from build123d import *

# Parameters (mm, degrees)
ESQUISSE1_W             = 30
ESQUISSE1_H             = 290
BOSS_EXTRU_1_DEPTH      = 5
ESQUISSE1_6_W           = 5
ESQUISSE1_6_H           = 8
ENL_V_MAT_EXTRU_1_DEPTH = 5
ESQUISSE1_7_W           = 5
ESQUISSE1_7_H           = 15
ESQUISSE1_7_H_2         = 8
ENL_V_MAT_EXTRU_2_DEPTH = 5


with BuildPart() as part:
    # Esquisse1 → Boss.-Extru.1 (new body)
    with BuildSketch(Plane.XY):
        with Locations((-15, 145)):
            Rectangle(ESQUISSE1_W, ESQUISSE1_H)
    extrude(amount=BOSS_EXTRU_1_DEPTH)

    # Esquisse1<6> → Enlèv. mat.-Extru.1 (cut)
    with BuildSketch(Plane.XY):
        with Locations((-2.5, 286)):
            Rectangle(ESQUISSE1_6_W, ESQUISSE1_6_H)
    extrude(amount=ENL_V_MAT_EXTRU_1_DEPTH, mode=Mode.SUBTRACT)

    # Esquisse1<7> → Enlèv. mat.-Extru.2 (cut)
    with BuildSketch(Plane.XY):
        with Locations((-21.11, 25)):
            Rectangle(ESQUISSE1_7_W, ESQUISSE1_7_H)
        with Locations((-21.11, 83)):
            Rectangle(ESQUISSE1_7_W, ESQUISSE1_7_H)
        with Locations((-21.11, 141)):
            Rectangle(ESQUISSE1_7_W, ESQUISSE1_7_H)
        with Locations((-21.11, 199)):
            Rectangle(ESQUISSE1_7_W, ESQUISSE1_7_H)
        with Locations((-21.11, 257)):
            Rectangle(ESQUISSE1_7_W, ESQUISSE1_7_H)
        with Locations((-27.5, 286)):
            Rectangle(ESQUISSE1_7_W, ESQUISSE1_7_H_2)
    extrude(amount=ENL_V_MAT_EXTRU_2_DEPTH, mode=Mode.SUBTRACT)


solid = part.part
Build history of the part. All positions in model axes, mm. A direction names the side the tool comes from. Coordinates: 2 decimals unless noted, no trailing zeros. Order: outer loops, then holes, each group sorted by start corner. A loop starts at its lowest first (then second) coordinate and runs counter-clockwise, first axis right, second up. Notation, with made-up numbers: (5, 81) -> (22, 81) arc R11 ccw to (22, 94) -> close; hole circle Ø3 at (22, 44). An arc over 180 degrees is marked (long way). One line per item, written item: value.
(1) Slice it at B-B, the plane z = 3.25. List the corners of the cut face in (x, y), plus the area to 4 significant figures.
Checked values:
outline: (-30, 0) -> (0, 0) -> (0, 282) -> (-5, 282) -> (-5, 290) -> (-25, 290) -> (-25, 282) -> (-30, 282) -> close; hole (-23.61, 17.5) -> (-18.61, 17.5) -> (-18.61, 32.5) -> (-23.61, 32.5) -> close; hole (-23.61, 75.5) -> (-18.61, 75.5) -> (-18.61, 90.5) -> (-23.61, 90.5) -> close; hole (-23.61, 133.5) -> (-18.61, 133.5) -> (-18.61, 148.5) -> (-23.61, 148.5) -> close; hole (-23.61, 191.5) -> (-18.61, 191.5) -> (-18.61, 206.5) -> (-23.61, 206.5) -> close; hole (-23.61, 249.5) -> (-18.61, 249.5) -> (-18.61, 264.5) -> (-23.61, 264.5) -> close
area: 8,245 mm2
(2) Drop flat-ended pins along their axis: pin 1 Ø1.5 at (x, z) = (-20.5, 1.5) entering from -Y; pin 2 Ø2.5 at (x, z) = (-2.5, 2.5) entering from +Y. Give the stop position or say it passes through.
Checked values:
pin 1: y = 0
pin 2: y = 282
(3) Tool access for faces 4 (the flat face through (-25, 286, 2)), 5 (the flat face through (-18.61, 199, 2)), 6 (the flat face through (0, 139, 2)): list every direction of +Z, -Z, +X, -X, +Y, -Y with a clear straight run to the whole face (end or side of a thin tool).
Checked values:
face 4: +Z, -Z, -X, +Y
face 5: +Z, -Z
face 6: +Z, -Z, +X, +Y, -Y
(4) Probe line 1 (Y direction, x = -20, z = 0.45); line 2 (X direction, y = 88, z = 1.3); line 3 (Y direction, x = -2.5, z = 3.4). List the from-to ranges inside material, lowest first. Write a range as [from, to].
Checked values:
line 1: [0, 17.5], [32.5, 75.5], [90.5, 133.5], [148.5, 191.5], [206.5, 249.5], [264.5, 290]
line 2: [-30, -23.61], [-18.61, 0]
line 3: [0, 282]
(5) Slice it at A-A, the plane y = 203. List the corners of the cut face in (x, z), plus the area to 3 significant figures.
Checked values:
outline: (-30, 0) -> (-23.61, 0) -> (-23.61, 5) -> (-30, 5) -> close; (-18.61, 0) -> (0, 0) -> (0, 5) -> (-18.61, 5) -> close
area: 125 mm2
(6) Mould opens along X. For faces 1 (the flat face through (-18.61, 83, 2)), 2 (the flat face through (-3, 282, 2)), 3 (the flat face through (-5, 286, 2)) say: pulls with the +X half, pulls with the -X half, needs draft (parallel to the pull), parting line crosses it, or undercut.
Checked values:
face 1: undercut
face 2: needs draft
face 3: pulls with the +X half
